from build123d import *

# Parameters (mm, degrees)
SKETCH3_R           = 22.5
BOSS_EXTRUDE1_DEPTH = 10
SKETCH4_R           = 11
BOSS_EXTRUDE2_DEPTH = 8.5
SKETCH5_R           = 2
CUT_EXTRUDE1_DEPTH  = 37.806928696


with BuildPart() as part:
    # Sketch3 → Boss-Extrude1 (new body)
    with BuildSketch(Plane(origin=(0, 0, 0), x_dir=(0, 0, -1), z_dir=(1, 0, 0))):
        Circle(SKETCH3_R)
    extrude(amount=BOSS_EXTRUDE1_DEPTH)

    # Sketch4 → Boss-Extrude2 (add)
    with BuildSketch(Plane(origin=(10, 0, 0), x_dir=(0, 0, -1), z_dir=(1, 0, 0))):
        Circle(SKETCH4_R)
    extrude(amount=BOSS_EXTRUDE2_DEPTH)

    # Sketch5 → Cut-Extrude1 (cut, through all)
    with BuildSketch(Plane(origin=(18.5, 0, 0), x_dir=(0, 0, -1), z_dir=(1, 0, 0))):
        with Locations((0, 8)):
            Circle(SKETCH5_R)
        with Locations((8, 0)):
            Circle(SKETCH5_R)
        with Locations((0, -8)):
            Circle(SKETCH5_R)
        with Locations((-8, 0)):
            Circle(SKETCH5_R)
    extrude(amount=-CUT_EXTRUDE1_DEPTH, mode=Mode.SUBTRACT)


solid = part.part
Check sheet for the modelled part. Datum: model origin and axes. Units: mm. A direction names the side the tool comes from. Round coordinates to 2 decimals unless told otherwise and drop trailing zeros. Loops run counter-clockwise (first coordinate to the right, second up) from the corner with the lowest first, then second, coordinate; pieces in that order, holes last. Notation, with made-up numbers: M 76,-22.75 L 131,-22.75 A11 ccw 131,-2.75 Z; hole C 26,75.25 d11. An arc over 180 degrees is marked long. One line per question, with ' | ' between items. Start each with the question number.
Item 1: Section check A-A (z = 0). Record the boundary of the cut face in (x, y), and give its area (3 significant figures).
Item 2: Section check D-D (x = 12.75). Record the boundary of the cut face in (y, z).
Item 3: Gauge pin test, flat ends, axial feed: pin 1 Ø8 at (y, z) = (-17.5, -11.5) entering from +X; pin 2 Ø1 at (x, z) = (5.5, 6) entering from -Y; pin 3 Ø5 at (x, z) = (8, 0) entering from -Y; pin 4 Ø3 at (y, z) = (0, 8) entering from -X. Record the tip position at first contact, or that the pin passes through.
Item 4: Release check for a two-part mould opening along Z. For faces 3 (the face through (9, 0, -6)), 4 (the face through (14.19, -10.74, 2.38)), 5 (the face through (9, 10, 0)), 6 (the face through (18.5, 0, 0)) record: released by +Z, released by -Z, zero draft, split by the parting line, or undercut.
Item 5: Scan lines: probe 1 along Y at (x, z) = (13, 0); probe 2 along Y at (x, z) = (6.75, 0); probe 3 along Z at (x, y) = (4, -1). Record each from-to range of solid material in increasing order.
Item 6: Set-up check for faces 1 (the face through (4.93, -19.961, -10.382)), 2 (the face through (10, 5, -10)): record each of +Z, -Z, +X, -X, +Y, -Y from which the full face is reachable in a straight line by a thin tool's end or side.
Item 7: Section check C-C (y = -8). Record the boundary of the cut face in (x, z), and give its area (3 significant figures).
Worked out:
1) outline: M 0,-22.5 L 10,-22.5 L 10,-11 L 18.5,-11 L 18.5,-10 L 0,-10 Z; M 0,-6 L 18.5,-6 L 18.5,6 L 0,6 Z; M 0,10 L 18.5,10 L 18.5,11 L 10,11 L 10,22.5 L 0,22.5 Z | area: 489 mm^2
2) outline: C 0,0 d22; hole C -8,0 d4; hole C 0,-8 d4; hole C 0,8 d4; hole C 8,0 d4
3) pin 1: x = 10 | pin 2: y = -21.82 | pin 3: y = -22.5 | pin 4: through
4) face 3: undercut | face 4: split by the parting line | face 5: undercut | face 6: zero draft
5) probe 1: -11 to -10, -6 to 6, 10 to 11 | probe 2: -22.5 to -10, -6 to 6, 10 to 22.5 | probe 3: -22.48 to -9.73, -6.27 to 6.27, 9.73 to 22.48
6) face 1: +X, -X | face 2: +X
7) outline: M 0,-21.03 L 10,-21.03 L 10,-7.55 L 18.5,-7.55 L 18.5,-2 L 0,-2 Z; M 0,2 L 18.5,2 L 18.5,7.55 L 10,7.55 L 10,21.03 L 0,21.03 Z | area: 475 mm^2
